Study the drawing (mm; zero at the part's minimum x, y, z) and answer. A direction names the side the tool comes from. Give positions to 0.01 mm unless a question says otherwise; leave off trailing zeros. Write each loop counter-clockwise with the first axis right and the second up, starting at its lowest first coordinate (ties: lowest second). Pieces come first, ordered by that corner, then holes. Notation, with made-up numbers: (37, -30) - (96, -30) arc R13 cw to (96, -26) - close; hole circle Ø3 at (51, 66.5). An arc over 180 degrees is marked (long way). Write each question's results on one line, items separated by ' | '. Start each with the question number.
Q1. Flat-ended cylindrical pins translate along their axes: pin 1 Ø4.5 at (x, z) = (58.07, 18.345) entering from -Y; pin 2 Ø3 at (x, y) = (19, 18) entering from -Z. Find the tip coordinate at first contact, or state that the pin passes through.
Q2. Section C-C (x = 51.77) is taken. Determine the outline of the cut face in (y, z) (3 decimals).
Q3. For a pull along X with two mould halves and no side action, classify the marked faces 1, 2, 3 and 4 as pulls with the +X half, pulls with the -X half, needs draft (parallel to the pull), parting line crosses it, or undercut.
Q4. Section D-D (z = 7.5) is taken. Determine the outline of the cut face in (x, y).
Q5. For the marked faces 5 and 6, determine the directions among +Z, -Z, +X, -X, +Y, -Y from which every point of the face is accessible in a straight line to the end or side of a thin tool.
Q6. Section A-A (x = 24) is taken. Determine the outline of the cut face in (y, z), plus the area to 3 significant figures.
Q7. Section B-B (y = 84) is taken. Determine the outline of the cut face in (x, z).
Q8. Find the intervals of material crossed by probe 1 along X at (y, z) = (89.5, 16.5); probe 2 along Y at (x, z) = (52.5, 26.5); probe 3 along Z at (x, y) = (58, 1), in increasing order.
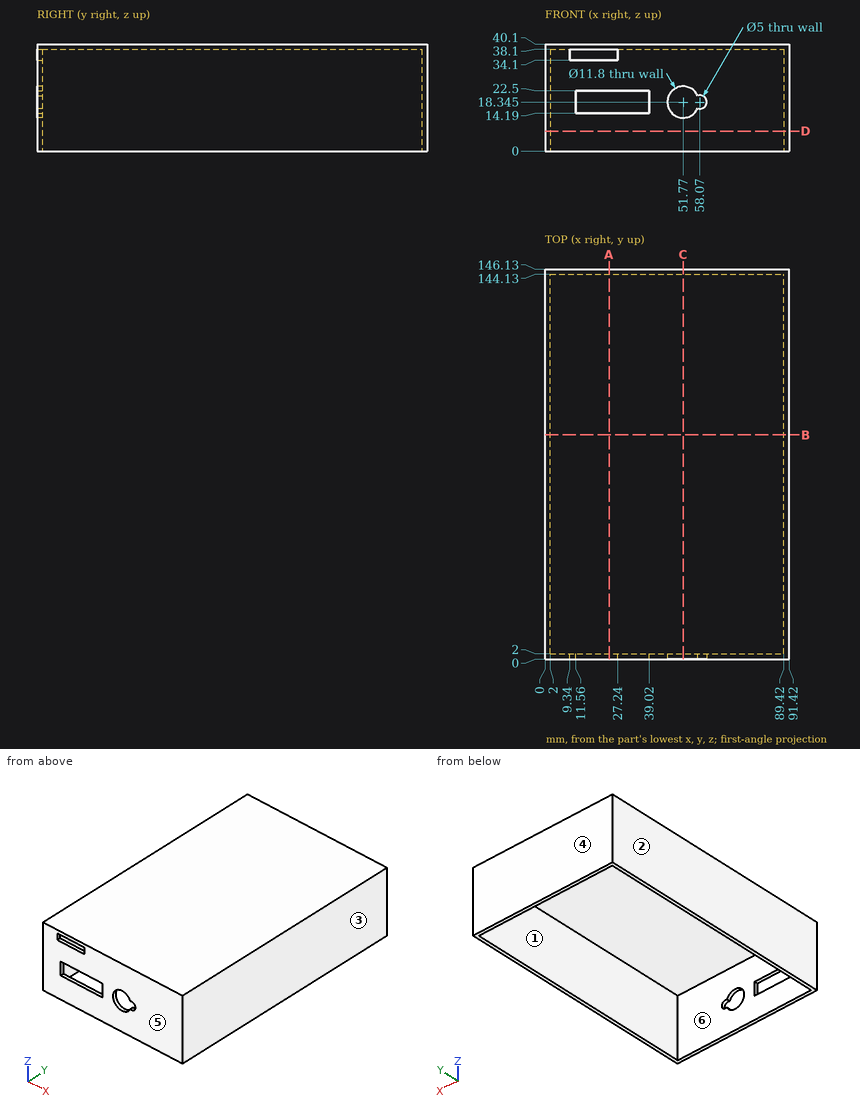
Answers below:
1) pin 1: stops at y = 144.13 | pin 2: stops at z = 38.1
2) outline: (0, 0) - (2, 0) - (2, 12.445) - (0, 12.445) - close; (0, 24.245) - (2, 24.245) - (2, 38.1) - (144.13, 38.1) - (144.13, 0) - (146.13, 0) - (146.13, 40.1) - (0, 40.1) - close
3) face 1: undercut | face 2: pulls with the -X half | face 3: pulls with the +X half | face 4: needs draft
4) outline: (0, 0) - (91.42, 0) - (91.42, 146.13) - (0, 146.13) - close; hole (2, 2) - (89.42, 2) - (89.42, 144.13) - (2, 144.13) - close
5) face 5: +Z, -Z, +X, -X, -Y | face 6: -Z
6) outline: (0, 0) - (2, 0) - (2, 14.19) - (0, 14.19) - close; (0, 22.5) - (2, 22.5) - (2, 34.1) - (0, 34.1) - close; (0, 38.1) - (144.13, 38.1) - (144.13, 0) - (146.13, 0) - (146.13, 40.1) - (0, 40.1) - close | area: 420 mm2
7) outline: (0, 0) - (2, 0) - (2, 38.1) - (89.42, 38.1) - (89.42, 0) - (91.42, 0) - (91.42, 40.1) - (0, 40.1) - close
8) probe 1: x = 0 to 2, 89.42 to 91.42 | probe 2: y = 0 to 2, 144.13 to 146.13 | probe 3: z = 0 to 15.85, 20.84 to 40.1
